Answer from the drawing. Dimensions are ordinates in mm from the lowest x, y and z of the part. A direction names the side the tool comes from. Give positions to 0.01 mm unless a question says otherwise; leave off trailing zeros. Order: outer loops, then holes, each group sorted by start corner. A loop starts at its lowest first (then second) coordinate and runs counter-clockwise, first axis right, second up.
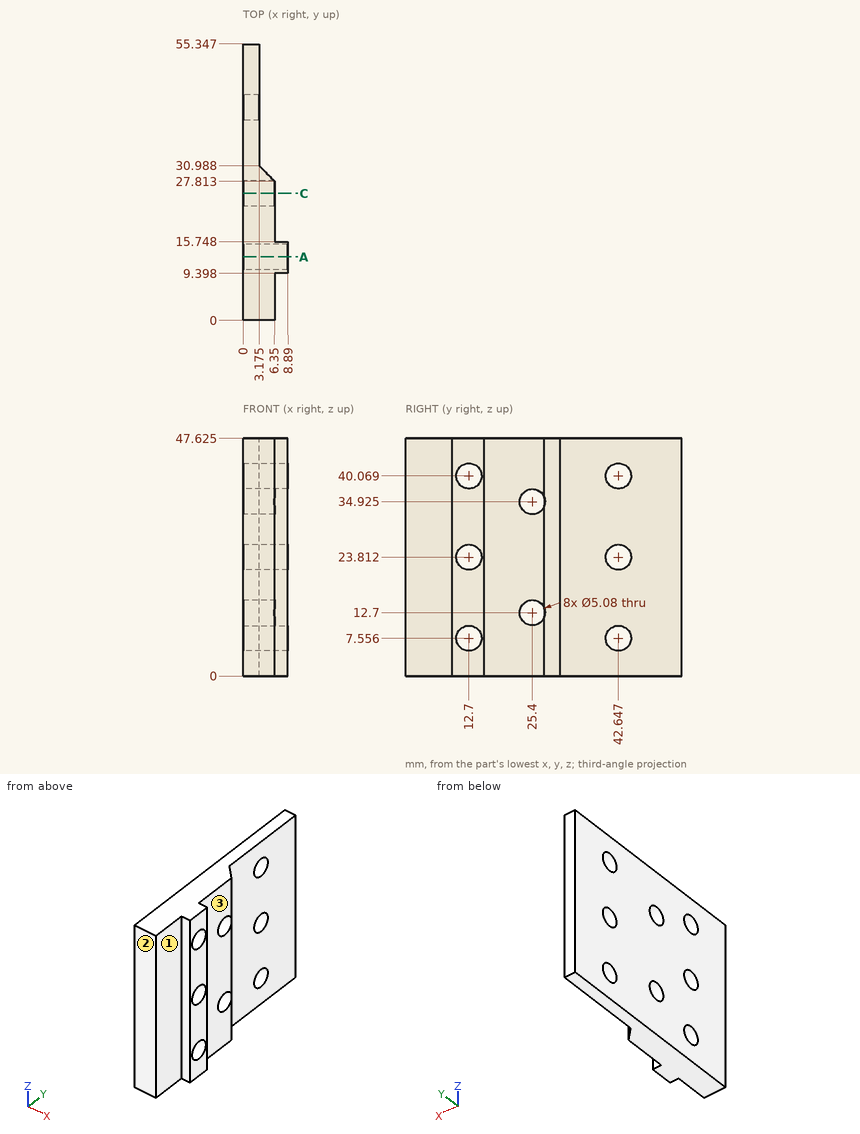
1. Which of the six approach directions +Z, -Z, +X, -X, +Y, -Y give full straight-line access (tool end or side, diameter ignored) to the marked faces 1, 2 and 3?
Findings below:
face 1: +Z, -Z, +X, -Y
face 2: +Z, -Z, +X, -X, -Y
face 3: +Z, -Z, +X, +Y
2. The part is cut by section C-C (y = 25.4). State how many separate pieces and enclosed holes the cut face has, then the cut area to 3 significant figures.
Findings below:
separate pieces: 3
enclosed holes: 0
area: 238 mm2
3. Straight lines are drawn through the part: probe 1 along Z at (x, y) = (1.5, 25) (1 decimal); probe 2 along X at (y, z) = (18, 4); probe 3 along Z at (x, y) = (1.75, 43) (1 decimal). For each, find the intervals that lie inside material, in ascending order.
Findings below:
probe 1: z = 0 to 10.2, 15.2 to 32.4, 37.4 to 47.6
probe 2: x = 0 to 6.35
probe 3: z = 0 to 5, 10.1 to 21.3, 26.3 to 37.6, 42.6 to 47.6
4. The part is cut by section A-A (y = 12.7). Write down the section's boundary in (x, z) (1 decimal).
Findings below:
outline: (0, 0) - (8.9, 0) - (8.9, 5) - (0, 5) - close; (0, 10.1) - (8.9, 10.1) - (8.9, 21.3) - (0, 21.3) - close; (0, 26.4) - (8.9, 26.4) - (8.9, 37.5) - (0, 37.5) - close; (0, 42.6) - (8.9, 42.6) - (8.9, 47.6) - (0, 47.6) - close
5. Given P1, Ø3, axis at x = 7.5, z = 20, coming from the -Y side; P2, Ø3.5, axis at y = 22.5, z = 29.5, coming from the +X side; P3, Ø7.5, axis at y = 48, z = 29, coming from the +X side (1 decimal), each flat-ended and moving along its own axis, determine where each tip first touches the part or whether it passes through.
Findings below:
P1: stops at y = 0
P2: stops at x = 6.35
P3: stops at x = 3.2
